from build123d import *

# Parameters (mm, degrees)
SKETCH1_R           = 5.95
BOSS_EXTRUDE2_DEPTH = 20
CUT_EXTRUDE1_DEPTH  = 41.875481649
CUT_EXTRUDE3_DEPTH  = 41.875481649
SKETCH10_R          = 3.8
CUT_EXTRUDE4_DEPTH  = 8
FILLET2_R           = 0.25


with BuildPart() as part:
    # Sketch1 → Boss-Extrude2 (new, symmetric)
    with BuildSketch(Plane.XY):
        Circle(SKETCH1_R)
    extrude(amount=BOSS_EXTRUDE2_DEPTH, both=True)

    # Sketch8 → Cut-Extrude1 (cut, through all)
    with BuildSketch(Plane.XY.offset(20)):
        Polygon((1.1, 1.05), (2.4, 1.05), (2.4, -1.05), (1.1, -1.05), (1.1, -2.35), (-1, -2.35), (-1, -1.05), (-2.3, -1.05), (-2.3, 1.05), (-1, 1.05), (-1, 2.35), (1.1, 2.35), align=None)
    extrude(amount=-CUT_EXTRUDE1_DEPTH, mode=Mode.SUBTRACT)

    # Sketch9 → Cut-Extrude3 (cut, through all)
    with BuildSketch(Plane.XY.offset(20)):
        with BuildLine():
            ThreePointArc((1.55, 5.744562647), (0, 5.95), (-1.55, 5.744562647))
            Line((-1.55, 5.744562647), (-1.55, 4.45))
            Line((-1.55, 4.45), (1.55, 4.45))
            Line((1.55, 4.45), (1.55, 5.744562647))
        make_face()
        with BuildLine():
            ThreePointArc((5.95, 0), (5.898417065, 0.781777543), (5.744562647, 1.55))
            Line((5.744562647, 1.55), (4.45, 1.55))
            Line((4.45, 1.55), (4.45, -1.55))
            Line((4.45, -1.55), (5.744562647, -1.55))
            ThreePointArc((5.744562647, -1.55), (5.898417065, -0.781777543), (5.95, 0))
        make_face()
        with BuildLine():
            Line((-4.45, 1.55), (-5.744562647, 1.55))
            ThreePointArc((-5.744562647, 1.55), (-5.95, 0), (-5.744562647, -1.55))
            Line((-5.744562647, -1.55), (-4.45, -1.55))
            Line((-4.45, -1.55), (-4.45, 1.55))
        make_face()
        with BuildLine():
            Line((-1.55, -4.45), (-1.55, -5.744562647))
            ThreePointArc((-1.55, -5.744562647), (0, -5.95), (1.55, -5.744562647))
            Line((1.55, -5.744562647), (1.55, -4.45))
            Line((1.55, -4.45), (-1.55, -4.45))
        make_face()
    extrude(amount=-CUT_EXTRUDE3_DEPTH, mode=Mode.SUBTRACT)

    # Sketch10 → Cut-Extrude4 (cut)
    with BuildSketch(Plane.XY.offset(20)):
        Circle(SKETCH10_R)
    cut_extrude4 = extrude(amount=-CUT_EXTRUDE4_DEPTH, mode=Mode.SUBTRACT)

    # Mirror1: Cut-Extrude4 across plane
    add(cut_extrude4.mirror(Plane.XY), mode=Mode.SUBTRACT)

    # Fillet2
    fillet2_edges = [part.edges().sort_by_distance(p)[0] for p in [
        (1.1, -1.05, 0),
        (1.1, 1.05, 0),
        (-1, 1.05, 0),
        (-1, -1.05, 0),
    ]]
    fillet(fillet2_edges, radius=FILLET2_R)


solid = part.part
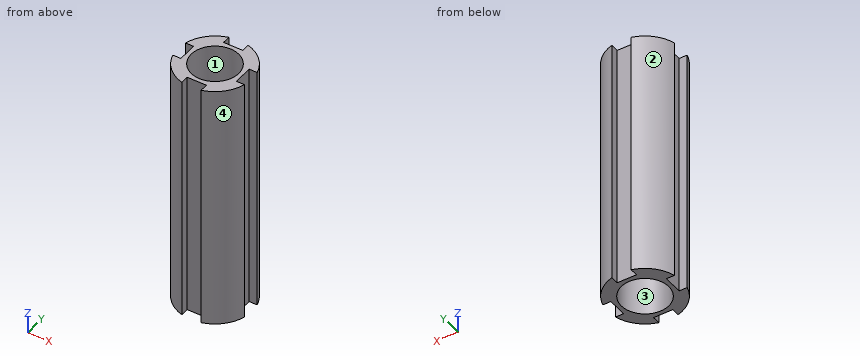
Geometry check sheet. Reference: the model listing, model coordinates, mm. Face numbers are marked on the shaded views. Give positions to 0.01 mm unless a question says otherwise; leave off trailing zeros. Loops run counter-clockwise (first coordinate to the right, second up) from the corner with the lowest first, then second, coordinate; pieces in that order, holes last. Notation, with made-up numbers: M 24,33.5 L 39,33.5 A22 ccw 39,69.5 Z; hole C -13.5,12 d2. An arc over 180 degrees is marked long. Write each question's results on one line, items separated by ' | '.
1) Thickness scan on line 1 (Y direction, x = 0, z = -17); line 2 (X direction, y = -1, z = -0.5); line 3 (Y direction, x = -1.25, z = 6). Record the ranges inside material, lowest first.
Answers follow:
line 1: -4.45 to -3.8, 3.8 to 4.45 | line 2: -4.45 to -2.3, 2.4 to 4.45 | line 3: -4.45 to -1.05, 1.05 to 4.45
2) Section check C-C, the plane y = 0. Record the boundary of the cut face in (x, z).
Answers follow:
outline: M -4.45,-20 L -3.8,-20 L -3.8,-12 L -2.3,-12 L -2.3,12 L -3.8,12 L -3.8,20 L -4.45,20 Z; M 2.4,-12 L 3.8,-12 L 3.8,-20 L 4.45,-20 L 4.45,20 L 3.8,20 L 3.8,12 L 2.4,12 Z
3) Section check A-A, the plane x = 0. Record the boundary of the cut face in (y, z), plus the area to 3 significant figures.
Answers follow:
outline: M -4.45,-20 L -3.8,-20 L -3.8,-12 L -2.35,-12 L -2.35,12 L -3.8,12 L -3.8,20 L -4.45,20 Z; M 2.35,-12 L 3.8,-12 L 3.8,-20 L 4.45,-20 L 4.45,20 L 3.8,20 L 3.8,12 L 2.35,12 Z | area: 122 mm2
4) Release check for a two-part mould opening along Y. For the marked faces 1, 2, 3 and 4 record: +Y half, -Y half, draft (parallel to the pull), parting line (faces both ways), or undercut.
Answers follow:
face 1: undercut | face 2: +Y half | face 3: undercut | face 4: -Y half
5) Section check D-D, the plane z = 16.5. Record the boundary of the cut face in (x, y).
Answers follow:
outline: M -5.74,-1.55 A5.95 ccw -1.55,-5.74 L -1.55,-4.45 L 1.55,-4.45 L 1.55,-5.74 A5.95 ccw 5.74,-1.55 L 4.45,-1.55 L 4.45,1.55 L 5.74,1.55 A5.95 ccw 1.55,5.74 L 1.55,4.45 L -1.55,4.45 L -1.55,5.74 A5.95 ccw -5.74,1.55 L -4.45,1.55 L -4.45,-1.55 Z; hole C 0,0 d7.6
6) Gauge pin test, flat ends, axial feed: pin 1 (1 mm diameter, centred on y = -5.5, z = -3.5, fed in from +X); pin 2 (0.5 mm diameter, centred on y = -2, z = 3, fed in from +X); pin 3 (3 mm diameter, centred on x = 0, z = 10.5, fed in from -Y). Record the tip position at first contact, or that the pin passes through.
Answers follow:
pin 1: x = 3.23 | pin 2: x = 5.69 | pin 3: y = -4.45
